Verification items for the finished model (mm, model axes). A direction names the side the tool comes from. Give positions to 0.01 mm unless a question says otherwise; leave off trailing zeros. Loops run counter-clockwise (first coordinate to the right, second up) from the corner with the lowest first, then second, coordinate; pieces in that order, holes last. Notation, with made-up numbers: (19, 42.5) - (66, 42.5) arc R22 cw to (66, 52.5) - close; hole circle Ø10 at (57.5, 30). An arc over 180 degrees is marked (long way). Answer in a Markdown table with one row per item.
```python
from build123d import *
from build123d.topology import SkipClean

# Parameters (mm, degrees)
SKETCH_1_R                        = 17
SKETCH_1_R_2                      = 6.5
EXTRUDE_2_DEPTH                   = 35
SKETCH_3_W                        = 33.795275063
SKETCH_3_H                        = 34.72803434
SKETCH_3_R                        = 13
EXTRUDE_7_DEPTH                   = 45
SKETCH_4_R                        = 6.5
CUT_EXTRUDE_1_DEPTH               = 60.489495005
SKETCH_12_R                       = 2
CUT_EXTRUDE_11_DEPTH              = 45
SKETCH_15_R                       = 2
CUT_EXTRUDE_12_DEPTH              = 45
FILLET_4_R                        = 10
SKETCH_20_R                       = 13
CUT_EXTRUDE_18_DEPTH              = 31
EXTRUDE_START                     = 1
SKETCH_25_R                       = 13
EXTRUDE_10_DEPTH                  = 1
SKETCH_26_R                       = 11.25
CUT_EXTRUDE_19_DEPTH              = 7.5
SKETCH_36_R                       = 4.5
SKETCH_36_R_2                     = 2
EXTRUDE_17_DEPTH                  = 15
EXTRUDE_17_DIRECTION_2_REACH      = 73.369
EXTRUDE_17_DIRECTION_2_END_RADIUS = 17
EXTRUDE_START_2                   = 3.5
EXTRUDE_18_DEPTH                  = 3.5
EXTRUDE_START_3                   = 12
SKETCH_41_R                       = 4.5
EXTRUDE_19_DEPTH                  = 12


with BuildPart() as part:
    # Эскиз1 → Бобышка-Вытянуть2 (new body)
    with BuildSketch(Plane.XY):
        Circle(SKETCH_1_R)
        Circle(SKETCH_1_R_2, mode=Mode.SUBTRACT)
    extrude(amount=EXTRUDE_2_DEPTH)

    # Эскиз3 → Бобышка-Вытянуть7 (add)
    with BuildSketch(Plane(origin=(0, 45, 0), x_dir=(1, 0, 0), z_dir=(0, 1, 0))):
        with Locations((0.102362468, -17.511098906)):
            Rectangle(SKETCH_3_W, SKETCH_3_H)
        with Locations(Location((0, -17.5, 0), (0, 0, 270))):
            Circle(SKETCH_3_R, mode=Mode.SUBTRACT)
    extrude(amount=-EXTRUDE_7_DEPTH)

    # Эскиз4 → Вырез-Вытянуть1 (cut, through all)
    with BuildSketch(Plane(origin=(0, 0, 0), x_dir=(-1, 0, 0), z_dir=(0, 0, -1))):
        with Locations(Location((0, 0, 0), (0, 0, 180))):
            Circle(SKETCH_4_R)
    extrude(amount=-CUT_EXTRUDE_1_DEPTH, mode=Mode.SUBTRACT)

    # Эскиз12 → Вырез-Вытянуть11 (cut)
    with BuildSketch(Plane(origin=(0, 0, 0), x_dir=(-1, 0, 0), z_dir=(0, 0, -1))):
        with Locations((0, 23)):
            Circle(SKETCH_12_R)
    extrude(amount=-CUT_EXTRUDE_11_DEPTH, mode=Mode.SUBTRACT)

    # Эскиз15 → Вырез-Вытянуть12 (cut)
    with BuildSketch(Plane.ZY.offset(16.795275063)):
        with Locations((17.5, 33)):
            Circle(SKETCH_15_R)
    extrude(amount=-CUT_EXTRUDE_12_DEPTH, mode=Mode.SUBTRACT)

    # Скругление4
    # the kernel refuses this fillet: 10 mm, written as the material it takes off along each edge
    with BuildSketch(Plane(origin=(-16.795275063, 70, 34.875116076), x_dir=(1, 0, 0), z_dir=(0, -1, 0))) as fillet_4_piece_1_section:
        with BuildLine():
            CenterArc((FILLET_4_R, -FILLET_4_R), FILLET_4_R, 90, 90)
            Line((0, -FILLET_4_R), (0, 0))
            Line((0, 0), (FILLET_4_R, 0))
        make_face()
    fillet_4_piece_1 = extrude(amount=92.369651061, mode=Mode.PRIVATE)
    fillet_4_piece_1 = fillet_4_piece_1 - Plane(origin=(0, 0, 32.54483178), x_dir=(1, 0, 0), z_dir=(0, 0, -1)) * Cylinder(17, 225, mode=Mode.PRIVATE)
    add(fillet_4_piece_1, mode=Mode.SUBTRACT)
    with BuildSketch(Plane(origin=(17, 70, 0.147081736), x_dir=(0, 0, 1), z_dir=(0, -1, 0))) as fillet_4_piece_2_section:
        with BuildLine():
            CenterArc((FILLET_4_R, FILLET_4_R), FILLET_4_R, 180, 90)
            Line((0, FILLET_4_R), (0, 0))
            Line((0, 0), (FILLET_4_R, 0))
        make_face()
    fillet_4_piece_2 = extrude(amount=95, mode=Mode.PRIVATE)
    fillet_4_piece_2 = fillet_4_piece_2 - Plane(origin=(0, 0, 2.486350956), x_dir=(1, 0, 0), z_dir=(0, 0, -1)) * Cylinder(17, 230, mode=Mode.PRIVATE)
    add(fillet_4_piece_2, mode=Mode.SUBTRACT)
    with BuildSketch(Plane(origin=(17, 70, 34.875116076), x_dir=(0, 0, -1), z_dir=(0, -1, 0))) as fillet_4_piece_3_section:
        with BuildLine():
            CenterArc((FILLET_4_R, -FILLET_4_R), FILLET_4_R, 90, 90)
            Line((0, -FILLET_4_R), (0, 0))
            Line((0, 0), (FILLET_4_R, 0))
        make_face()
    fillet_4_piece_3 = extrude(amount=95, mode=Mode.PRIVATE)
    fillet_4_piece_3 = fillet_4_piece_3 - Plane(origin=(0, 0, 32.535846855), x_dir=(1, 0, 0), z_dir=(0, 0, -1)) * Cylinder(17, 230, mode=Mode.PRIVATE)
    add(fillet_4_piece_3, mode=Mode.SUBTRACT)
    with BuildSketch(Plane(origin=(-16.795275063, 70, 0.147081736), x_dir=(0, 0, 1), z_dir=(0, -1, 0))) as fillet_4_piece_4_section:
        with BuildLine():
            CenterArc((FILLET_4_R, -FILLET_4_R), FILLET_4_R, 90, 90)
            Line((0, -FILLET_4_R), (0, 0))
            Line((0, 0), (FILLET_4_R, 0))
        make_face()
    fillet_4_piece_4 = extrude(amount=92.369651061, mode=Mode.PRIVATE)
    fillet_4_piece_4 = fillet_4_piece_4 - Plane(origin=(0, 0, 2.477367304), x_dir=(1, 0, 0), z_dir=(0, 0, -1)) * Cylinder(17, 225, mode=Mode.PRIVATE)
    add(fillet_4_piece_4, mode=Mode.SUBTRACT)

    # Эскиз20 → Вырез-Вытянуть18 (cut)
    with SkipClean():  # the faces are left unmerged after this step: merging them gives an invalid solid
        with BuildSketch(Plane(origin=(0, 45, 0), x_dir=(1, 0, 0), z_dir=(0, 1, 0))):
            with Locations(Location((0, -17.5, 0), (0, 0, 270))):
                Circle(SKETCH_20_R)
        extrude(amount=-CUT_EXTRUDE_18_DEPTH, mode=Mode.SUBTRACT)

    # Эскиз25 → Бобышка-Вытянуть10 (add)
    with BuildSketch(Plane(origin=(0, 14, 0), x_dir=(1, 0, 0), z_dir=(0, 1, 0)).offset(EXTRUDE_START)):
        with Locations(Location((0, -17.5, 0), (0, 0, 270))):
            Circle(SKETCH_25_R)
    extrude(amount=-EXTRUDE_10_DEPTH)

    # Эскиз26 → Вырез-Вытянуть19 (cut)
    with BuildSketch(Plane(origin=(0, 0, 0), x_dir=(-1, 0, 0), z_dir=(0, 0, -1))):
        Circle(SKETCH_26_R)
    extrude(amount=-CUT_EXTRUDE_19_DEPTH, mode=Mode.SUBTRACT)

    # Эскиз36 → Бобышка-Вытянуть17 (add)
    with BuildSketch(Plane(origin=(14.722431864, -8.5, 0), x_dir=(0, 0, -1), z_dir=(0.8660254037844346, -0.5000000000000071, 0))):
        with Locations(Location((-17.511098906, 0, 0), (0, 0, 270))):
            Circle(SKETCH_36_R)
        with Locations(Location((-17.511098906, 0, 0), (0, 0, 90))):
            Circle(SKETCH_36_R_2, mode=Mode.SUBTRACT)
    extrude(amount=EXTRUDE_17_DEPTH)

    # Бобышка-Вытянуть17 direction 2: up to this cylinder (the profile starts outside it)
    with SkipClean():  # the faces are left unmerged after this step: merging them gives an invalid solid
        extrude_17_direction_2_end = Plane(origin=(0, 0, 17.511099), z_dir=(0, 0, -1)) * Cylinder(EXTRUDE_17_DIRECTION_2_END_RADIUS, 181.738, mode=Mode.PRIVATE)
        # Эскиз36 → Бобышка-Вытянуть17 direction 2 (add, up to the surface)
        with BuildSketch(Plane(origin=(14.722431864, -8.5, 0), x_dir=(0, 0, -1), z_dir=(0.8660254037844346, -0.5000000000000071, 0)), mode=Mode.PRIVATE) as extrude_17_direction_2_sk1:
            with Locations(Location((-17.511098906, 0, 0), (0, 0, 270))):
                Circle(SKETCH_36_R)
            with Locations(Location((-17.511098906, 0, 0), (0, 0, 90))):
                Circle(SKETCH_36_R_2, mode=Mode.SUBTRACT)
        extrude_17_direction_2_tool1 = extrude(extrude_17_direction_2_sk1.sketch, amount=-EXTRUDE_17_DIRECTION_2_REACH, mode=Mode.PRIVATE) - extrude_17_direction_2_end
        add(extrude_17_direction_2_tool1.solids().sort_by_distance((16.908792, -4.713113, 17.511099))[0])
        add(extrude_17_direction_2_tool1.solids().sort_by_distance((16.908792, -4.713113, 17.511099))[1])

    # Эскиз40 → Бобышка-Вытянуть18 (add)
    with BuildSketch(Plane(origin=(27.712812921, -16, 0), x_dir=(0, 0, -1), z_dir=(0.8660254037844346, -0.5000000000000071, 0)).offset(EXTRUDE_START_2)):
        with BuildLine():
            Line((-15.998598906, 2.619726846), (-13.852269687, 2.619726846))
            ThreePointArc((-13.852269687, 2.619726846), (-22.011098906, 0), (-13.852269687, -2.619726846))
            Line((-13.852269687, -2.619726846), (-15.998598906, -2.619726846))
            Line((-15.998598906, -2.619726846), (-19.023598906, -2.619726846))
            Line((-19.023598906, -2.619726846), (-20.536098906, 0))
            Line((-20.536098906, 0), (-19.023598906, 2.619726846))
            Line((-19.023598906, 2.619726846), (-15.998598906, 2.619726846))
        make_face()
    extrude(amount=-EXTRUDE_18_DEPTH)

    # Эскиз41 → Бобышка-Вытянуть19 (add)
    with BuildSketch(Plane(origin=(30.743901834, -17.75, 0), x_dir=(0, 0, -1), z_dir=(0.8660254037844346, -0.5000000000000071, 0)).offset(EXTRUDE_START_3)):
        with Locations(Location((-17.511098906, 0, 0), (0, 0, 270))):
            Circle(SKETCH_41_R)
    extrude(amount=-EXTRUDE_19_DEPTH)


solid = part.part
```
Q1. Tool access check on faces 1 (the face through (30.76, -17.72, 16.72)), 2 (the face through (11.07, 12.9, 17.38)), 3 (the face through (-13.79, 28.82, 32.02)). Record the directions out of +Z, -Z, +X, -X, +Y, -Y that give a thin tool (end or side, any length) a straight path to the whole face; none if there is none.
Completed:
| item | result |
|---|---|
| face 1 | -Z |
| face 2 | none |
| face 3 | +Z, -X, +Y |
Q2. Draft check along Y on faces 4 (the face through (14.892, 31.048, 17.066)), 5 (the face through (41.168, -23.695, 17.448)), 6 (the face through (7, 0, 35)). Enter one of: +Y half, -Y half, draft (parallel to the pull), parting line (faces both ways), or undercut.
Completed:
| item | result |
|---|---|
| face 4 | undercut |
| face 5 | -Y half |
| face 6 | draft |
Q3. Sectioned sample at C-C (y = 33). Record the cut outline in (x, z), and give its area (3 significant figures).
Completed:
| item | result |
|---|---|
| outline | (-16.8, 10.15) arc R10 ccw to (-6.8, 0.15) - (7, 0.15) arc R10 ccw to (17, 10.15) - (17, 15.5) - (12.85, 15.5) arc R13 cw to (-12.85, 15.5) - (-16.8, 15.5) - close; (-16.8, 19.5) - (-12.85, 19.5) arc R13 cw to (12.85, 19.5) - (17, 19.5) - (17, 24.88) arc R10 ccw to (7, 34.88) - (-6.8, 34.88) arc R10 ccw to (-16.8, 24.88) - close |
| area | 525 mm^2 |
Q4. Go/stop test with flat-tipped pins: P1, Ø1, axis at x = -12, z = 18.5, coming from the -Y side; P2, Ø7.5, axis at y = 25.5, z = 21, coming from the +X side; P3, Ø12, axis at y = 30, z = 17, coming from the -X side; P4, Ø12, axis at x = -9, z = 9.5, coming from the +Y side. Record where each tip stops, or that it passes through.
Completed:
| item | result |
|---|---|
| P1 | y = -12.52 |
| P2 | x = 17 |
| P3 | x = -16.8 |
| P4 | y = 45 |
Q5. Thickness scan on line 1 (Y direction, x = 0, z = 2.2); line 2 (Y direction, x = -0.5, z = 13); line 3 (X direction, y = 29, z = 17). Record the ranges inside material, lowest first.
Completed:
| item | result |
|---|---|
| line 1 | -17 to -11.25, 11.25 to 21, 25 to 45 |
| line 2 | -16.99 to -6.48, 6.48 to 15 |
| line 3 | -16.8 to -12.99, 12.99 to 17 |
Q6. Sectioned sample at A-A (y = 23). Record the cut outline in (x, z), and give its area (3 significant figures).
Completed:
| item | result |
|---|---|
| outline | (-16.8, 10.15) arc R10 ccw to (-6.8, 0.15) - (-2, 0.15) - (-2, 4.65) arc R13 cw to (-2, 30.35) - (-2, 34.88) - (-6.8, 34.88) arc R10 ccw to (-16.8, 24.88) - close; (2, 0.15) - (7, 0.15) arc R10 ccw to (17, 10.15) - (17, 24.88) arc R10 ccw to (7, 34.88) - (2, 34.88) - (2, 30.35) arc R13 cw to (2, 4.65) - close |
| area | 522 mm^2 |
Q7. Sectioned sample at D-D (z = 32). Record the cut outline in (x, y).
Completed:
| item | result |
|---|---|
| outline | (-13.81, 9.91) arc R17 ccw (long way) to (14.02, 9.62) - (14.02, 45) - (-13.81, 45) - close; hole circle Ø13 at (0, 0); hole circle Ø4 at (0, 23) |
Q8. Sectioned sample at B-B (x = -3). Record the cut outline in (y, z).
Completed:
| item | result |
|---|---|
| outline | (-16.73, 0) - (-10.84, 0) - (-10.84, 7.5) - (-5.77, 7.5) - (-5.77, 35) - (-16.73, 35) - close; (5.77, 7.5) - (10.84, 7.5) - (10.84, 0) - (16.73, 0) - (16.73, 0.15) - (45, 0.15) - (45, 4.85) - (15, 4.85) - (15, 30.15) - (45, 30.15) - (45, 34.88) - (16.73, 34.88) - (16.73, 35) - (5.77, 35) - close |
